Read the model definition and answer for the solid it produces. Units are mm, in the model's axes. A direction names the side the tool comes from. Coordinates: 2 decimals unless noted, no trailing zeros. Loops run counter-clockwise (first coordinate to the right, second up) from the corner with the lowest first, then second, coordinate; pieces in that order, holes last. Notation, with made-up numbers: (22.25, -33.5) -> (33.25, -33.5) arc R19 ccw to (33.25, -13.5) -> close; hole circle Ø2 at (2.5, 14.5). An arc over 180 degrees is marked (long way). Answer as a JSON object with one key per item and string values. Group by question number.
1) Which of the six approach directions +Z, -Z, +X, -X, +Y, -Y give full straight-line access (tool end or side, diameter ignored) to faces 1 (the face through (10.13, -45.16, 46.53)), 2 (the face through (-103, 55, 47)), 3 (the face through (-93.5, 50.4, 45))?
2) Section D-D, the plane y = -36.5 is taken. Give the vertices of the cut face in (x, z).
3) Flat-ended cylindrical pins translate along their axes: P1, Ø1.2, axis at x = -103, z = 46, coming from the -Y side; P2, Ø3.5, axis at y = 50, z = 40, coming from the +X side; P3, Ø2.5, axis at y = -50, z = 41.5, coming from the -X side; P4, Ø4, axis at x = 40, y = 36.5, coming from the +Z side. Find the tip coordinate at first contact, or state that the pin passes through.
4) Section A-A, the plane y = 10.5 is taken. Give the vertices of the cut face in (x, z).
5) Section B-B, the plane x = -30.5 is taken. Give the vertices of the cut face in (y, z), plus the area to 3 significant figures.
6) Consider probe 1 along Y at (x, z) = (-95, 47.4); probe 2 along Y at (x, z) = (-90, 44.65); probe 3 along Y at (x, z) = (-44.5, 46.5). Determine where each line is inside the solid, lowest interval first. Write a range as [from, to].
7) Determine the mould class of faces 4 (the face through (-102, -55, 47)), 5 (the face through (12.12, 11.01, 46.53)), 6 (the face through (-20, 51.5, 41)) for opening direction Y: released by +Y, released by -Y, zero draft, split by the parting line, or undercut.
8) Section C-C, the plane z = 38.75 is taken. Give the vertices of the cut face in (x, y).
from build123d import *

# Parameters (mm, degrees)
MAIN_PROFILE_SKETCH_R       = 3.4
MAIN_PROFILE_SKETCH_R_2     = 1.7
MAIN_EXTRUSION_DEPTH        = 3.5
DETAIL_PROFILE_2_SKETCH_R   = 5.3
DETAIL_PROFILE_2_SKETCH_R_2 = 1.7
DETAIL_EXTRUSION_2_DEPTH    = 0.5
DETAIL_PROFILE_3_SKETCH_W   = 85.5
DETAIL_PROFILE_3_SKETCH_H   = 3
DETAIL_EXTRUSION_3_DEPTH    = 0.2
DETAIL_PROFILE_4_SKETCH_W   = 85.5
DETAIL_PROFILE_4_SKETCH_H   = 3
DETAIL_EXTRUSION_4_DEPTH    = 7.8


with BuildPart() as part:
    # Main Profile Sketch → Main Extrusion (new body)
    with BuildSketch(Plane.XY.offset(48.5)):
        with BuildLine():
            Line((-85.126602828, 55), (55, 55))
            Line((55, 55), (55, -55))
            Line((55, -55), (-85.126602828, -55))
            ThreePointArc((-85.126602828, -55), (-90, -57.5), (-94.873397172, -55))
            Line((-94.873397172, -55), (-110, -55))
            Line((-110, -55), (-110, 55))
            Line((-110, 55), (-94.873397172, 55))
            ThreePointArc((-94.873397172, 55), (-90, 57.5), (-85.126602828, 55))
        make_face()
        with Locations((-90, -51.5)):
            Circle(MAIN_PROFILE_SKETCH_R, mode=Mode.SUBTRACT)
        with Locations((-95, -45)):
            Circle(MAIN_PROFILE_SKETCH_R_2, mode=Mode.SUBTRACT)
        with Locations((-85.5, -43.5)):
            Circle(MAIN_PROFILE_SKETCH_R_2, mode=Mode.SUBTRACT)
        with Locations((-95, -36.5)):
            Circle(MAIN_PROFILE_SKETCH_R_2, mode=Mode.SUBTRACT)
        with Locations((-44.5, -43.5)):
            Circle(MAIN_PROFILE_SKETCH_R_2, mode=Mode.SUBTRACT)
        with Locations((-30.5, -43.5)):
            Circle(MAIN_PROFILE_SKETCH_R_2, mode=Mode.SUBTRACT)
        with Locations((-98.5, -27)):
            Circle(MAIN_PROFILE_SKETCH_R_2, mode=Mode.SUBTRACT)
        with Locations((-85.5, -10.5)):
            Circle(MAIN_PROFILE_SKETCH_R_2, mode=Mode.SUBTRACT)
        with Locations((-44.5, -10.5)):
            Circle(MAIN_PROFILE_SKETCH_R_2, mode=Mode.SUBTRACT)
        with Locations((-30.5, -10.5)):
            Circle(MAIN_PROFILE_SKETCH_R_2, mode=Mode.SUBTRACT)
        with Locations((10.5, -43.5)):
            Circle(MAIN_PROFILE_SKETCH_R_2, mode=Mode.SUBTRACT)
        with Locations((24.5, -43.5)):
            Circle(MAIN_PROFILE_SKETCH_R_2, mode=Mode.SUBTRACT)
        with Locations((40, -36.5)):
            Circle(MAIN_PROFILE_SKETCH_R_2, mode=Mode.SUBTRACT)
        with Locations((10.5, -10.5)):
            Circle(MAIN_PROFILE_SKETCH_R_2, mode=Mode.SUBTRACT)
        with Locations((24.5, -10.5)):
            Circle(MAIN_PROFILE_SKETCH_R_2, mode=Mode.SUBTRACT)
        with Locations((-85.5, 10.5)):
            Circle(MAIN_PROFILE_SKETCH_R_2, mode=Mode.SUBTRACT)
        with Locations((-98.5, 27)):
            Circle(MAIN_PROFILE_SKETCH_R_2, mode=Mode.SUBTRACT)
        with Locations((-44.5, 10.5)):
            Circle(MAIN_PROFILE_SKETCH_R_2, mode=Mode.SUBTRACT)
        with Locations((-30.5, 10.5)):
            Circle(MAIN_PROFILE_SKETCH_R_2, mode=Mode.SUBTRACT)
        with Locations((-102, 34.5)):
            Circle(MAIN_PROFILE_SKETCH_R_2, mode=Mode.SUBTRACT)
        with Locations((-95, 36.5)):
            Circle(MAIN_PROFILE_SKETCH_R_2, mode=Mode.SUBTRACT)
        with Locations((-95, 45)):
            Circle(MAIN_PROFILE_SKETCH_R_2, mode=Mode.SUBTRACT)
        with Locations((-102, 51.5)):
            Circle(MAIN_PROFILE_SKETCH_R_2, mode=Mode.SUBTRACT)
        with Locations((-90, 51.5)):
            Circle(MAIN_PROFILE_SKETCH_R, mode=Mode.SUBTRACT)
        with Locations((-85.5, 43.5)):
            Circle(MAIN_PROFILE_SKETCH_R_2, mode=Mode.SUBTRACT)
        with Locations((-44.5, 43.5)):
            Circle(MAIN_PROFILE_SKETCH_R_2, mode=Mode.SUBTRACT)
        with Locations((-30.5, 43.5)):
            Circle(MAIN_PROFILE_SKETCH_R_2, mode=Mode.SUBTRACT)
        with Locations((10.5, 10.5)):
            Circle(MAIN_PROFILE_SKETCH_R_2, mode=Mode.SUBTRACT)
        with Locations((24.5, 10.5)):
            Circle(MAIN_PROFILE_SKETCH_R_2, mode=Mode.SUBTRACT)
        with Locations((10.5, 43.5)):
            Circle(MAIN_PROFILE_SKETCH_R_2, mode=Mode.SUBTRACT)
        with Locations((40, 36.5)):
            Circle(MAIN_PROFILE_SKETCH_R_2, mode=Mode.SUBTRACT)
        with Locations((24.5, 43.5)):
            Circle(MAIN_PROFILE_SKETCH_R_2, mode=Mode.SUBTRACT)
    extrude(amount=-MAIN_EXTRUSION_DEPTH)

    # Detail Profile 2 Sketch → Detail Extrusion 2 (add)
    with BuildSketch(Plane.XY.offset(45)):
        with BuildLine():
            Line((-85.126602828, 55), (55, 55))
            Line((55, 55), (55, -55))
            Line((55, -55), (-85.126602828, -55))
            ThreePointArc((-85.126602828, -55), (-90, -57.5), (-94.873397172, -55))
            Line((-94.873397172, -55), (-110, -55))
            Line((-110, -55), (-110, 55))
            Line((-110, 55), (-94.873397172, 55))
            ThreePointArc((-94.873397172, 55), (-90, 57.5), (-85.126602828, 55))
        make_face()
        with Locations((-90, -51.5)):
            Circle(DETAIL_PROFILE_2_SKETCH_R, mode=Mode.SUBTRACT)
        with Locations((-95, -45)):
            Circle(DETAIL_PROFILE_2_SKETCH_R_2, mode=Mode.SUBTRACT)
        with Locations((-85.5, -43.5)):
            Circle(DETAIL_PROFILE_2_SKETCH_R_2, mode=Mode.SUBTRACT)
        with Locations((-95, -36.5)):
            Circle(DETAIL_PROFILE_2_SKETCH_R_2, mode=Mode.SUBTRACT)
        with Locations((-44.5, -43.5)):
            Circle(DETAIL_PROFILE_2_SKETCH_R_2, mode=Mode.SUBTRACT)
        with Locations((-30.5, -43.5)):
            Circle(DETAIL_PROFILE_2_SKETCH_R_2, mode=Mode.SUBTRACT)
        with Locations((-98.5, -27)):
            Circle(DETAIL_PROFILE_2_SKETCH_R_2, mode=Mode.SUBTRACT)
        with Locations((-85.5, -10.5)):
            Circle(DETAIL_PROFILE_2_SKETCH_R_2, mode=Mode.SUBTRACT)
        with Locations((-44.5, -10.5)):
            Circle(DETAIL_PROFILE_2_SKETCH_R_2, mode=Mode.SUBTRACT)
        with Locations((-30.5, -10.5)):
            Circle(DETAIL_PROFILE_2_SKETCH_R_2, mode=Mode.SUBTRACT)
        with Locations((10.5, -43.5)):
            Circle(DETAIL_PROFILE_2_SKETCH_R_2, mode=Mode.SUBTRACT)
        with Locations((24.5, -43.5)):
            Circle(DETAIL_PROFILE_2_SKETCH_R_2, mode=Mode.SUBTRACT)
        with Locations((40, -36.5)):
            Circle(DETAIL_PROFILE_2_SKETCH_R_2, mode=Mode.SUBTRACT)
        with Locations((10.5, -10.5)):
            Circle(DETAIL_PROFILE_2_SKETCH_R_2, mode=Mode.SUBTRACT)
        with Locations((24.5, -10.5)):
            Circle(DETAIL_PROFILE_2_SKETCH_R_2, mode=Mode.SUBTRACT)
        with Locations((-85.5, 10.5)):
            Circle(DETAIL_PROFILE_2_SKETCH_R_2, mode=Mode.SUBTRACT)
        with Locations((-98.5, 27)):
            Circle(DETAIL_PROFILE_2_SKETCH_R_2, mode=Mode.SUBTRACT)
        with Locations((-44.5, 10.5)):
            Circle(DETAIL_PROFILE_2_SKETCH_R_2, mode=Mode.SUBTRACT)
        with Locations((-30.5, 10.5)):
            Circle(DETAIL_PROFILE_2_SKETCH_R_2, mode=Mode.SUBTRACT)
        with Locations((-102, 34.5)):
            Circle(DETAIL_PROFILE_2_SKETCH_R_2, mode=Mode.SUBTRACT)
        with Locations((-95, 36.5)):
            Circle(DETAIL_PROFILE_2_SKETCH_R_2, mode=Mode.SUBTRACT)
        with Locations((-95, 45)):
            Circle(DETAIL_PROFILE_2_SKETCH_R_2, mode=Mode.SUBTRACT)
        with Locations((-102, 51.5)):
            Circle(DETAIL_PROFILE_2_SKETCH_R_2, mode=Mode.SUBTRACT)
        with Locations((-90, 51.5)):
            Circle(DETAIL_PROFILE_2_SKETCH_R, mode=Mode.SUBTRACT)
        with Locations((-85.5, 43.5)):
            Circle(DETAIL_PROFILE_2_SKETCH_R_2, mode=Mode.SUBTRACT)
        with Locations((-44.5, 43.5)):
            Circle(DETAIL_PROFILE_2_SKETCH_R_2, mode=Mode.SUBTRACT)
        with Locations((-30.5, 43.5)):
            Circle(DETAIL_PROFILE_2_SKETCH_R_2, mode=Mode.SUBTRACT)
        with Locations((10.5, 10.5)):
            Circle(DETAIL_PROFILE_2_SKETCH_R_2, mode=Mode.SUBTRACT)
        with Locations((24.5, 10.5)):
            Circle(DETAIL_PROFILE_2_SKETCH_R_2, mode=Mode.SUBTRACT)
        with Locations((10.5, 43.5)):
            Circle(DETAIL_PROFILE_2_SKETCH_R_2, mode=Mode.SUBTRACT)
        with Locations((40, 36.5)):
            Circle(DETAIL_PROFILE_2_SKETCH_R_2, mode=Mode.SUBTRACT)
        with Locations((24.5, 43.5)):
            Circle(DETAIL_PROFILE_2_SKETCH_R_2, mode=Mode.SUBTRACT)
    extrude(amount=-DETAIL_EXTRUSION_2_DEPTH)

    # Detail Profile 3 Sketch → Detail Extrusion 3 (add)
    with BuildSketch(Plane.XY.offset(44.5)):
        with BuildLine():
            Line((-107, -48.5), (-94.369210455, -48.5))
            ThreePointArc((-94.369210455, -48.5), (-95.061956905, -49.929461145), (-95.3, -51.5))
            Line((-95.3, -51.5), (-107, -51.5))
            Line((-107, -51.5), (-107, -48.5))
        make_face()
        with BuildLine():
            Line((-85.630789545, -48.5), (-85, -48.5))
            Line((-85, -48.5), (-85, -49.742160417))
            ThreePointArc((-85, -49.742160417), (-85.274403026, -49.100263923), (-85.630789545, -48.5))
        make_face()
        with Locations((-19.25, -50)):
            Rectangle(DETAIL_PROFILE_3_SKETCH_W, DETAIL_PROFILE_3_SKETCH_H)
        with BuildLine():
            Line((-107, 51.5), (-105.7, 51.5))
            ThreePointArc((-105.7, 51.5), (-105.294151704, 49.81519599), (-104.165640783, 48.5))
            Line((-104.165640783, 48.5), (-107, 48.5))
            Line((-107, 48.5), (-107, 51.5))
        make_face()
        with BuildLine():
            Line((-98.3, 51.5), (-95.3, 51.5))
            ThreePointArc((-95.3, 51.5), (-95.061956905, 49.929461145), (-94.369210455, 48.5))
            Line((-94.369210455, 48.5), (-99.834359217, 48.5))
            ThreePointArc((-99.834359217, 48.5), (-98.705848296, 49.81519599), (-98.3, 51.5))
        make_face()
        with BuildLine():
            Line((-85, 49.742160417), (-85, 48.5))
            Line((-85, 48.5), (-85.630789545, 48.5))
            ThreePointArc((-85.630789545, 48.5), (-85.274403026, 49.100263923), (-85, 49.742160417))
        make_face()
        with Locations((-19.25, 50)):
            Rectangle(DETAIL_PROFILE_3_SKETCH_W, DETAIL_PROFILE_3_SKETCH_H)
    extrude(amount=-DETAIL_EXTRUSION_3_DEPTH)

    # Detail Profile 4 Sketch → Detail Extrusion 4 (add)
    with BuildSketch(Plane.XY.offset(44.3)):
        with BuildLine():
            Line((-107, -48.5), (-91.374772708, -48.5))
            ThreePointArc((-91.374772708, -48.5), (-92.777296342, -49.717691096), (-93.3, -51.5))
            Line((-93.3, -51.5), (-107, -51.5))
            Line((-107, -51.5), (-107, -48.5))
        make_face()
        with BuildLine():
            Line((-85, -48.5), (-85, -51.5))
            Line((-85, -51.5), (-86.7, -51.5))
            ThreePointArc((-86.7, -51.5), (-87.222703658, -49.717691096), (-88.625227292, -48.5))
            Line((-88.625227292, -48.5), (-85, -48.5))
        make_face()
        with Locations((-19.25, -50)):
            Rectangle(DETAIL_PROFILE_4_SKETCH_W, DETAIL_PROFILE_4_SKETCH_H)
        with BuildLine():
            Line((-107, 51.5), (-105.7, 51.5))
            ThreePointArc((-105.7, 51.5), (-105.294151704, 49.81519599), (-104.165640783, 48.5))
            Line((-104.165640783, 48.5), (-107, 48.5))
            Line((-107, 48.5), (-107, 51.5))
        make_face()
        with BuildLine():
            Line((-98.3, 51.5), (-93.3, 51.5))
            ThreePointArc((-93.3, 51.5), (-92.777296342, 49.717691096), (-91.374772708, 48.5))
            Line((-91.374772708, 48.5), (-99.834359217, 48.5))
            ThreePointArc((-99.834359217, 48.5), (-98.705848296, 49.81519599), (-98.3, 51.5))
        make_face()
        with BuildLine():
            Line((-86.7, 51.5), (-85, 51.5))
            Line((-85, 51.5), (-85, 48.5))
            Line((-85, 48.5), (-88.625227292, 48.5))
            ThreePointArc((-88.625227292, 48.5), (-87.222703658, 49.717691096), (-86.7, 51.5))
        make_face()
        with Locations((-19.25, 50)):
            Rectangle(DETAIL_PROFILE_4_SKETCH_W, DETAIL_PROFILE_4_SKETCH_H)
    extrude(amount=-DETAIL_EXTRUSION_4_DEPTH)


solid = part.part
Determined:
{
 "1": {"face 1": "+Z, -Z", "face 2": "+Z, -Z, -X, +Y", "face 3": "none"},
 "2": {"outline": "(-110, 44.5) -> (-96.7, 44.5) -> (-96.7, 48.5) -> (-110, 48.5) -> close; (-93.3, 44.5) -> (38.3, 44.5) -> (38.3, 48.5) -> (-93.3, 48.5) -> close; (41.7, 44.5) -> (55, 44.5) -> (55, 48.5) -> (41.7, 48.5) -> close"},
 "3": {"P1": "y = -55", "P2": "x = 23.5", "P3": "x = -107", "P4": "z = 48.5"},
 "4": {"outline": "(-110, 44.5) -> (-87.2, 44.5) -> (-87.2, 48.5) -> (-110, 48.5) -> close; (-83.8, 44.5) -> (-46.2, 44.5) -> (-46.2, 48.5) -> (-83.8, 48.5) -> close; (-42.8, 44.5) -> (-32.2, 44.5) -> (-32.2, 48.5) -> (-42.8, 48.5) -> close; (-28.8, 44.5) -> (8.8, 44.5) -> (8.8, 48.5) -> (-28.8, 48.5) -> close; (12.2, 44.5) -> (22.8, 44.5) -> (22.8, 48.5) -> (12.2, 48.5) -> close; (26.2, 44.5) -> (55, 44.5) -> (55, 48.5) -> (26.2, 48.5) -> close"},
 "5": {"outline": "(-55, 44.5) -> (-51.5, 44.5) -> (-51.5, 36.5) -> (-48.5, 36.5) -> (-48.5, 44.5) -> (-45.2, 44.5) -> (-45.2, 48.5) -> (-55, 48.5) -> close; (-41.8, 44.5) -> (-12.2, 44.5) -> (-12.2, 48.5) -> (-41.8, 48.5) -> close; (-8.8, 44.5) -> (8.8, 44.5) -> (8.8, 48.5) -> (-8.8, 48.5) -> close; (12.2, 44.5) -> (41.8, 44.5) -> (41.8, 48.5) -> (12.2, 48.5) -> close; (45.2, 44.5) -> (48.5, 44.5) -> (48.5, 36.5) -> (51.5, 36.5) -> (51.5, 44.5) -> (55, 44.5) -> (55, 48.5) -> (45.2, 48.5) -> close", "area": "434 mm²"},
 "6": {"probe 1": "[-55, -46.7], [-43.3, -38.2], [-34.8, 34.8], [38.2, 43.3], [46.7, 55]", "probe 2": "[-57.5, -56.8], [-46.2, 46.2], [56.8, 57.5]", "probe 3": "[-55, -45.2], [-41.8, -12.2], [-8.8, 8.8], [12.2, 41.8], [45.2, 55]"},
 "7": {"face 4": "released by -Y", "face 5": "undercut", "face 6": "released by +Y"},
 "8": {"outline": "(-107, -51.5) -> (-93.3, -51.5) arc R3.3 cw to (-91.37, -48.5) -> (-107, -48.5) -> close; (-107, 48.5) -> (-104.17, 48.5) arc R3.7 cw to (-105.7, 51.5) -> (-107, 51.5) -> close; (-99.83, 48.5) -> (-91.37, 48.5) arc R3.3 cw to (-93.3, 51.5) -> (-98.3, 51.5) arc R3.7 cw to start; (-88.63, -48.5) arc R3.3 cw to (-86.7, -51.5) -> (-85, -51.5) -> (-85, -48.5) -> close; (-88.63, 48.5) -> (-85, 48.5) -> (-85, 51.5) -> (-86.7, 51.5) arc R3.3 cw to start; (-62, -51.5) -> (23.5, -51.5) -> (23.5, -48.5) -> (-62, -48.5) -> close; (-62, 48.5) -> (23.5, 48.5) -> (23.5, 51.5) -> (-62, 51.5) -> close"}
}
